Part model, mm, in its own coordinate system. Face numbers are marked on the shaded views. A direction names the side the tool comes from. Round coordinates to 2 decimals unless told otherwise and drop trailing zeros. Loops run counter-clockwise (first coordinate to the right, second up) from the corner with the lowest first, then second, coordinate; pieces in that order, holes last.
(1) Cut at B-B on z = 83. List the corners of the cut face in (x, y), then the cut area to 3 significant figures.
(2) Cut at C-C on y = 12.7. List the corners of the cut face in (x, z).
(3) Tool access for the marked faces 1 and 2: list every direction of +Z, -Z, +X, -X, +Y, -Y with a clear straight run to the whole face (end or side of a thin tool).
(4) Flat gauge pin, fed straight in: pin 1 (1 mm diameter, centred on y = 4.5, z = 109, fed in from -X). Where does the tip first touch, or does it go through?
(5) Probe probe 1 along Y at (x, z) = (10.5, 110.5); probe 2 along Z at (x, y) = (5.5, 16.5); probe 3 along Z at (x, y) = (12, 12.5). List the from-to ranges inside material, lowest first.
(6) Mould opens along Y. For the marked faces 3, 4, 5 and 6 say: +Y half, -Y half, draft (parallel to the pull), parting line (faces both ways), or undercut.
(7) Cut at A-A on x = 5.5. List the corners of the cut face in (y, z).
from build123d import *

# Parameters (mm, degrees)
SKETCH1_W           = 152.4
SKETCH1_H           = 25.4
BOSS_EXTRUDE1_DEPTH = 12.7
CUT_EXTRUDE2_REACH  = 156.654


with BuildPart() as part:
    # Sketch1 → Boss-Extrude1 (new body)
    with BuildSketch(Plane(origin=(0, 0, 0), x_dir=(0, 0, -1), z_dir=(1, 0, 0))):
        with Locations((-76.2, 12.7)):
            Rectangle(SKETCH1_W, SKETCH1_H)
    extrude(amount=BOSS_EXTRUDE1_DEPTH)

    # Sketch3 → Cut-Extrude2 (cut, up to next)
    with BuildSketch(Plane(origin=(12.7, 2.360975137, 0), x_dir=(0, 0, -1), z_dir=(1, 0, 0)), mode=Mode.PRIVATE) as cut_extrude2_sk1:
        with BuildLine():
            Line((-136.033448355, 19.329867732), (-16.366551645, 19.329867732))
            ThreePointArc((-16.366551645, 19.329867732), (-7.375708776, 10.339024863), (-16.366551645, 1.348181995))
            Line((-16.366551645, 1.348181995), (-136.033448355, 1.348181995))
            ThreePointArc((-136.033448355, 1.348181995), (-145.024291224, 10.339024863), (-136.033448355, 19.329867732))
        make_face()
    cut_extrude2_tool1 = extrude(cut_extrude2_sk1.sketch, amount=-CUT_EXTRUDE2_REACH, mode=Mode.PRIVATE) & part.part
    add(cut_extrude2_tool1.solids().sort_by_distance((12.7, 12.7, 76.2))[0], mode=Mode.SUBTRACT)


solid = part.part
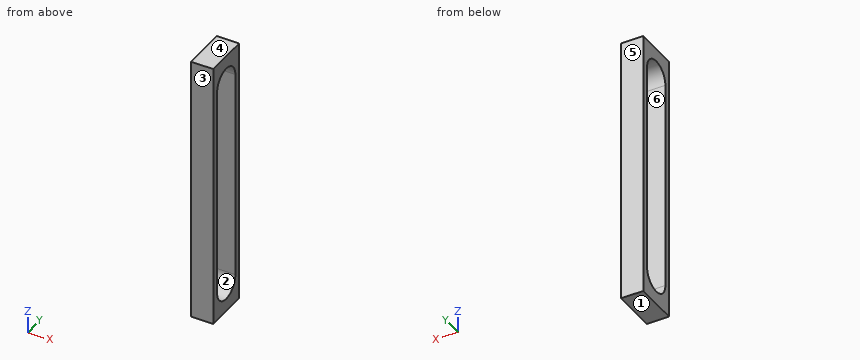
Final values:
1. outline: (0, 0) - (12.7, 0) - (12.7, 3.71) - (0, 3.71) - close; (0, 21.69) - (12.7, 21.69) - (12.7, 25.4) - (0, 25.4) - close
1. area: 94.2 mm2
2. outline: (0, 0) - (12.7, 0) - (12.7, 7.38) - (0, 7.38) - close; (0, 145.02) - (12.7, 145.02) - (12.7, 152.4) - (0, 152.4) - close
3. face 1: -Z, +X, -X, +Y, -Y
3. face 2: +X, -X
4. pin 1: passes through
5. probe 1: y = 0 to 3.71, 21.69 to 25.4
5. probe 2: z = 0 to 8.22, 144.18 to 152.4
5. probe 3: z = 0 to 7.38, 145.02 to 152.4
6. face 3: -Y half
6. face 4: draft
6. face 5: +Y half
6. face 6: undercut
7. outline: (0, 0) - (25.4, 0) - (25.4, 152.4) - (0, 152.4) - close; hole (3.71, 16.37) arc R8.99 ccw to (21.69, 16.37) - (21.69, 136.03) arc R8.99 ccw to (3.71, 136.03) - close
